from build123d import *

# Parameters (mm, degrees)
SKETCH2_W                      = 95
SKETCH2_H                      = 63.5
BOSS_EXTRUDE1_DEPTH            = 8
M3_CLEARANCE_HOLE1_D           = 3.4
M3_CLEARANCE_HOLE1_CSINK_D     = 3.45
M3_CLEARANCE_HOLE1_CSINK_ANGLE = 90
CUT_EXTRUDE1_DEPTH             = 10
CUT_EXTRUDE2_DEPTH             = 2.4
FILLET2_R                      = 2


with BuildPart() as part:
    # Sketch2 → Boss-Extrude1 (new body)
    with BuildSketch(Plane(origin=(0, 0, 0), x_dir=(1, 0, 0), z_dir=(0, 1, 0))):
        Rectangle(SKETCH2_W, SKETCH2_H)
    extrude(amount=BOSS_EXTRUDE1_DEPTH)

    # M3 Clearance Hole1 (through all)
    with Locations(Plane(origin=(0, 8, 0), x_dir=(1, 0, 0), z_dir=(0, 1, 0))):
        with Locations((-40.666732268, 24.17), (-40.666732268, -24.17), (34.463267732, 24.17), (41.963267732, -24.17), (11.143267732, -19.17), (11.143267732, 8.85)):
            CounterSinkHole(M3_CLEARANCE_HOLE1_D / 2, M3_CLEARANCE_HOLE1_CSINK_D / 2, counter_sink_angle=M3_CLEARANCE_HOLE1_CSINK_ANGLE)

    # Sketch9 → Cut-Extrude1 (cut)
    with BuildSketch(Plane(origin=(0, 8, 0), x_dir=(1, 0, 0), z_dir=(0, 1, 0))):
        with BuildLine():
            Line((-34.974163292, 19.487383717), (-34.974163292, 22.75))
            ThreePointArc((-34.974163292, 22.75), (-34.095483636, 24.871320344), (-31.974163292, 25.75))
            Line((-31.974163292, 25.75), (-1.684765082, 25.75))
            ThreePointArc((-1.684765082, 25.75), (0.436555262, 24.871320344), (1.315234918, 22.75))
            Line((1.315234918, 22.75), (1.315234918, 7.055031971))
            ThreePointArc((1.315234918, 7.055031971), (2.193914574, 4.933711628), (4.315234918, 4.055031971))
            Line((4.315234918, 4.055031971), (17.971300546, 4.055031971))
            ThreePointArc((17.971300546, 4.055031971), (20.09262089, 4.933711628), (20.971300546, 7.055031971))
            Line((20.971300546, 7.055031971), (20.971300546, 16.428287462))
            ThreePointArc((20.971300546, 16.428287462), (21.849980203, 18.549607805), (23.971300546, 19.428287462))
            Line((23.971300546, 19.428287462), (38.5, 19.428287462))
            ThreePointArc((38.5, 19.428287462), (40.621320344, 18.549607805), (41.5, 16.428287462))
            Line((41.5, 16.428287462), (41.5, -14.560508757))
            ThreePointArc((41.5, -14.560508757), (40.621320344, -16.681829101), (38.5, -17.560508757))
            Line((38.5, -17.560508757), (37.647901029, -17.560508757))
            ThreePointArc((37.647901029, -17.560508757), (35.526580685, -18.439188414), (34.647901029, -20.560508757))
            Line((34.647901029, -20.560508757), (34.647901029, -22.75))
            ThreePointArc((34.647901029, -22.75), (33.769221372, -24.871320344), (31.647901029, -25.75))
            Line((31.647901029, -25.75), (23.971300546, -25.75))
            ThreePointArc((23.971300546, -25.75), (21.849980203, -24.871320344), (20.971300546, -22.75))
            Line((20.971300546, -22.75), (20.971300546, -18.118028913))
            ThreePointArc((20.971300546, -18.118028913), (20.09262089, -15.996708569), (17.971300546, -15.118028913))
            Line((17.971300546, -15.118028913), (4.315234918, -15.118028913))
            ThreePointArc((4.315234918, -15.118028913), (2.193914574, -15.996708569), (1.315234918, -18.118028913))
            Line((1.315234918, -18.118028913), (1.315234918, -22.75))
            ThreePointArc((1.315234918, -22.75), (0.436555262, -24.871320344), (-1.684765082, -25.75))
            Line((-1.684765082, -25.75), (-28.730080623, -25.75))
            ThreePointArc((-28.730080623, -25.75), (-30.851400966, -24.871320344), (-31.730080623, -22.75))
            Line((-31.730080623, -22.75), (-31.730080623, -22.252488185))
            ThreePointArc((-31.730080623, -22.252488185), (-32.608760279, -20.131167841), (-34.730080623, -19.252488185))
            Line((-34.730080623, -19.252488185), (-38.5, -19.252488185))
            ThreePointArc((-38.5, -19.252488185), (-40.621320344, -18.373808528), (-41.5, -16.252488185))
            Line((-41.5, -16.252488185), (-41.5, 13.487383717))
            ThreePointArc((-41.5, 13.487383717), (-40.621320344, 15.60870406), (-38.5, 16.487383717))
            Line((-38.5, 16.487383717), (-37.974163292, 16.487383717))
            ThreePointArc((-37.974163292, 16.487383717), (-35.852842949, 17.366063373), (-34.974163292, 19.487383717))
        make_face()
    extrude(amount=-CUT_EXTRUDE1_DEPTH, mode=Mode.SUBTRACT)

    # Sketch10 → Cut-Extrude2 (cut)
    with BuildSketch(Plane.XZ):
        Polygon((-41.401711603, 20.903023001), (-38.204936861, 21.900000725), (-37.469957526, 25.166977724), (-39.931752933, 27.436976999), (-43.128527675, 26.439999275), (-43.86350701, 23.173022276), align=None)
        Polygon((-41.973397742, -27.253173474), (-38.649958452, -26.843192232), (-37.343292978, -23.760018758), (-39.360066794, -21.086826526), (-42.683506084, -21.496807768), (-43.990171558, -24.579981242), align=None)
        Polygon((8.072719548, -10.186064064), (10.765059061, -12.177204763), (13.835607245, -10.841140699), (14.213815916, -7.513935936), (11.521476403, -5.522795237), (8.450928219, -6.858859301), align=None)
        Polygon((8.080180086, 17.816919291), (10.783526176, 15.84074793), (13.846613823, 17.193828639), (14.206355378, 20.523080709), (11.503009288, 22.49925207), (8.439921642, 21.146171361), align=None)
        Polygon((32.605291512, -26.95590339), (35.94694273, -27.172006301), (37.804918951, -24.386102911), (36.321243952, -21.38409661), (32.979592734, -21.167993699), (31.121616514, -23.953897089), align=None)
        Polygon((40.040474323, 21.428431318), (43.376139153, 21.13402772), (45.298932562, 23.875596402), (43.886061141, 26.911568682), (40.550396312, 27.20597228), (38.627602903, 24.464403598), align=None)
    extrude(amount=-CUT_EXTRUDE2_DEPTH, mode=Mode.SUBTRACT)

    # Fillet2
    fillet2_edges = [part.edges().sort_by_distance(p)[0] for p in [
        (47.5, 8, 0),
        (0, 8, -31.75),
        (-47.5, 8, 0),
        (0, 8, 31.75),
    ]]
    fillet(fillet2_edges, radius=FILLET2_R)


solid = part.part
Part model, mm, in its own coordinate system. A direction names the side the tool comes from. Coordinates: 2 decimals unless noted, no trailing zeros. Order: outer loops, then holes, each group sorted by start corner. A loop starts at its lowest first (then second) coordinate and runs counter-clockwise, first axis right, second up. Notation, with made-up numbers: M 55.25,3.25 L 104.25,3.25 A22 cw 104.25,28.25 Z; hole C 52,76.25 d6. An arc over 180 degrees is marked long. Use a Markdown table: item, result.
(1) Cut at A-A on x = -8. Write the cut outline in (y, z).
A:
| item | result |
|---|---|
| outline | M 0,-31.75 L 6,-31.75 A2 ccw 8,-29.75 L 8,-25.75 L 0,-25.75 Z; M 0,25.75 L 8,25.75 L 8,29.75 A2 ccw 6,31.75 L 0,31.75 Z |
(2) Cut at C-C on z = -8.85. Write the cut outline in (x, y) (3 decimals), then the cut area to 3 significant figures.
A:
| item | result |
|---|---|
| outline | M -47.5,0 L -41.5,0 L -41.5,8 L -45.5,8 A2 ccw -47.5,6 Z; M 1.315,0 L 8.225,0 L 8.225,2.4 L 9.443,2.4 L 9.443,7.975 L 9.418,8 L 1.315,8 Z; M 12.843,2.4 L 14.062,2.4 L 14.062,0 L 20.971,0 L 20.971,8 L 12.868,8 L 12.843,7.975 Z; M 41.5,0 L 47.5,0 L 47.5,6 A2 ccw 45.5,8 L 41.5,8 Z |
| area | 218 mm^2 |
(3) Pull direction X, two halves, no side cores. Call faces 3 (the flat face through (-38.34, 1.18, -22.44)), 4 (the flat face through (10, 0, -15)): released by +X, released by -X, zero draft, split by the parting line, or undercut.
A:
| item | result |
|---|---|
| face 3 | undercut |
| face 4 | zero draft |
(4) Probe L1, parallel to X at y = 4.5, z = -13.5; L2, parallel to Z at x = 25, y = 5.25; L3, parallel to Z at x = -21.5, y = 4. List the from-to ranges inside material, lowest first.
A:
| item | result |
|---|---|
| L1 | x = -47.5 to -41.5, 1.32 to 20.97, 41.5 to 47.5 |
| L2 | z = -31.75 to -19.43, 25.75 to 31.75 |
| L3 | z = -31.75 to -25.75, 25.75 to 31.75 |
(5) Tool access for faces 1 (the flat face through (32.064, 1.183, -22.541)), 2 (the flat face through (-37, 4, 19.252)): list every direction of +Z, -Z, +X, -X, +Y, -Y with a clear straight run to the whole face (end or side of a thin tool).
A:
| item | result |
|---|---|
| face 1 | -Y |
| face 2 | +Y, -Y |
(6) Flat gauge pins, fed straight in: pin 1 (3 mm diameter, centred on x = 41.96, z = 24.17, fed in from +Y); pin 2 (3 mm diameter, centred on x = 35.5, z = -23.5, fed in from -Y). Where does each tip first touch, or does it go through?
A:
| item | result |
|---|---|
| pin 1 | passes through |
| pin 2 | stops at y = 2.4 |
(7) Cut at D-D on y = 1.25. State how many separate pieces and enclosed holes the cut face has, then the cut area to 3 significant figures.
A:
| item | result |
|---|---|
| separate pieces | 1 |
| enclosed holes | 7 |
| area | 2,540 mm^2 |
(8) Cut at B-B on z = 12. Write the cut outline in (x, y).
A:
| item | result |
|---|---|
| outline | M -47.5,0 L -41.5,0 L -41.5,8 L -45.5,8 A2 ccw -47.5,6 Z; M 41.5,0 L 47.5,0 L 47.5,6 A2 ccw 45.5,8 L 41.5,8 Z |
